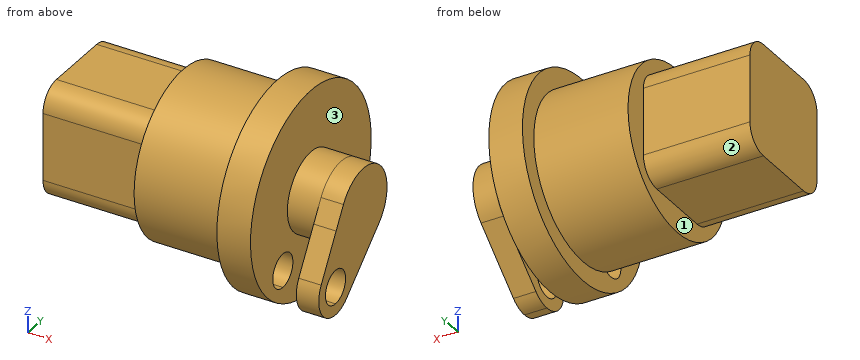
```python
from build123d import *

# Parameters (mm, degrees)
SKETCH2_R           = 9
BOSS_EXTRUDE1_DEPTH = 3
SKETCH2_4_R         = 7.3
BOSS_EXTRUDE2_DEPTH = 8.4
BOSS_EXTRUDE3_START = -8.4
SKETCH2_6_W         = 10
SKETCH2_6_H         = 10
BOSS_EXTRUDE3_DEPTH = 9.5
BOSS_EXTRUDE6_START = 3
SKETCH6_R           = 3.5
BOSS_EXTRUDE6_DEPTH = 2.7
BOSS_EXTRUDE7_START = 5.7
BOSS_EXTRUDE7_DEPTH = 2
CUT_EXTRUDE1_DEPTH  = 3
FILLET1_R           = 2


with BuildPart() as part:
    # Sketch2 → Boss-Extrude1 (new body)
    with BuildSketch(Plane(origin=(0, 0, 0), x_dir=(0, 0, -1), z_dir=(1, 0, 0))):
        Circle(SKETCH2_R)
    extrude(amount=BOSS_EXTRUDE1_DEPTH)

    # Sketch2<4> → Boss-Extrude2 (add)
    with BuildSketch(Plane(origin=(0, 0, 0), x_dir=(0, 0, -1), z_dir=(1, 0, 0))):
        Circle(SKETCH2_4_R)
    extrude(amount=-BOSS_EXTRUDE2_DEPTH)

    # Sketch2<6> → Boss-Extrude3 (add)
    with BuildSketch(Plane(origin=(0, 0, 0), x_dir=(0, 0, -1), z_dir=(1, 0, 0)).offset(BOSS_EXTRUDE3_START)):
        Rectangle(SKETCH2_6_W, SKETCH2_6_H)
    extrude(amount=-BOSS_EXTRUDE3_DEPTH)

    # Sketch6 → Boss-Extrude6 (add)
    with BuildSketch(Plane(origin=(0, 0, 0), x_dir=(0, 0, -1), z_dir=(1, 0, 0)).offset(BOSS_EXTRUDE6_START)):
        with Locations(Location((0, 0, 0), (0, 0, 180))):
            Circle(SKETCH6_R)
    extrude(amount=BOSS_EXTRUDE6_DEPTH)

    # Sketch6<4> → Boss-Extrude7 (add)
    with BuildSketch(Plane(origin=(0, 0, 0), x_dir=(0, 0, -1), z_dir=(1, 0, 0)).offset(BOSS_EXTRUDE7_START)):
        with BuildLine():
            ThreePointArc((6.861759117, -2.533034113), (4.954197643, -1.67824538), (3.064177772, -2.571150439))
            Line((3.064177772, -2.571150439), (3.830222216, -3.213938048))
            ThreePointArc((3.830222216, -3.213938048), (5.492319095, -2.768580532), (6.47928888, -4.178119463))
            ThreePointArc((6.47928888, -4.178119463), (6.388827811, -4.691149678), (6.128355545, -5.142300877))
            Line((6.128355545, -5.142300877), (6.894399988, -5.785088487))
            ThreePointArc((6.894399991, -5.785088484), (7.328520433, -5.033169819), (7.47928888, -4.178119463))
            ThreePointArc((7.47928888, -4.178119463), (7.3198204, -3.29953412), (6.861759117, -2.533034113))
        make_face()
        with BuildLine():
            Line((3.830222216, -3.213938048), (3.064177772, -2.571150439))
            ThreePointArc((3.064177772, -2.571150439), (2.513036454, -4.587507997), (3.6860836, -6.31765682))
            ThreePointArc((3.6860836, -6.31765682), (5.388677416, -6.644371889), (6.894399991, -5.785088484))
            Line((6.894399988, -5.785088487), (6.128355545, -5.142300877))
            ThreePointArc((6.128355545, -5.142300877), (4.015107466, -5.327186128), (3.830222216, -3.213938048))
        make_face()
        with BuildLine():
            ThreePointArc((3.5, 0), (3.288924173, -1.197070502), (2.681155551, -2.249756634))
            Line((2.681155551, -2.249756634), (3.064177772, -2.571150439))
            ThreePointArc((3.064177772, -2.571150439), (4.954197643, -1.67824538), (6.861759117, -2.533034113))
            Line((6.861759117, -2.533034113), (2.635458332, 2.303119489))
            ThreePointArc((2.635458332, 2.303119489), (3.276744128, 1.230019479), (3.5, 0))
        make_face()
        with BuildLine():
            Line((3.064177772, -2.571150439), (2.681155551, -2.249756634))
            ThreePointArc((2.681155551, -2.249756634), (1.479163916, -3.172077255), (0, -3.5))
            Line((0, -3.5), (0, -4.089669185))
            Line((0, -4.089669185), (3.6860836, -6.31765682))
            ThreePointArc((3.6860836, -6.31765682), (2.513036454, -4.587507997), (3.064177772, -2.571150439))
        make_face()
        with BuildLine():
            Line((0, -3.5), (0, 0))
            Line((0, 0), (2.681155551, -2.249756634))
            ThreePointArc((2.681155551, -2.249756634), (3.288924173, -1.197070502), (3.5, 0))
            ThreePointArc((3.5, 0), (3.276744128, 1.230019479), (2.635458332, 2.303119489))
            ThreePointArc((2.635458332, 2.303119489), (-2.681155551, 2.249756634), (-1.810487393, -2.9953523))
            ThreePointArc((-1.810487393, -2.9953523), (-0.939751816, -3.371478389), (0, -3.5))
        make_face()
        with BuildLine():
            Line((2.681155551, -2.249756634), (0, 0))
            Line((0, 0), (0, -3.5))
            ThreePointArc((0, -3.5), (1.479163916, -3.172077255), (2.681155551, -2.249756634))
        make_face()
        with BuildLine():
            Line((0, -4.089669185), (0, -3.5))
            ThreePointArc((0, -3.5), (-0.939751816, -3.371478389), (-1.810487393, -2.9953523))
            Line((-1.810487393, -2.9953523), (0, -4.089669185))
        make_face()
    extrude(amount=BOSS_EXTRUDE7_DEPTH)

    # Sketch6<5> → Cut-Extrude1 (cut)
    with BuildSketch(Plane(origin=(0, 0, 0), x_dir=(0, 0, -1), z_dir=(1, 0, 0))):
        with BuildLine():
            ThreePointArc((6.47928888, -4.178119463), (5.492319095, -2.768580532), (3.830222216, -3.213938048))
            Line((3.830222216, -3.213938048), (6.128355545, -5.142300877))
            ThreePointArc((6.128355545, -5.142300877), (6.388827811, -4.691149678), (6.47928888, -4.178119463))
        make_face()
        with BuildLine():
            Line((6.128355545, -5.142300877), (3.830222216, -3.213938048))
            ThreePointArc((3.830222216, -3.213938048), (4.015107466, -5.327186128), (6.128355545, -5.142300877))
        make_face()
    extrude(amount=CUT_EXTRUDE1_DEPTH, mode=Mode.SUBTRACT)

    # Fillet1
    fillet1_edges = [part.edges().sort_by_distance(p)[0] for p in [
        (-13.15, -5, 5),
        (-13.15, 5, 5),
        (-13.15, 5, -5),
        (-13.15, -5, -5),
    ]]
    fillet(fillet1_edges, radius=FILLET1_R)


solid = part.part
```
Verification items for the finished model (mm, model axes). Face numbers are marked on the shaded views. A direction names the side the tool comes from. Coordinates: 2 decimals unless noted, no trailing zeros. Loops run counter-clockwise (first coordinate to the right, second up) from the corner with the lowest first, then second, coordinate; pieces in that order, holes last. Notation, with made-up numbers: (54, 56.5) -> (70, 56.5) arc R25 ccw to (70, 73.5) -> close; hole circle Ø4 at (-19, 41). An arc over 180 degrees is marked (long way). Answer in a Markdown table with one row per item. Add a question column.
1. Material ranges on probe 1 along Z at (x, y) = (-11, 0.75); probe 2 along X at (y, z) = (-4.5, -1.25); probe 3 along X at (y, z) = (-1.5, 6.75), recorded low to high. Write a range as [from, to].
2. Section check B-B, the plane y = 4.5. Enter the section's corners in (x, z).
3. Access from +Z, -Z, +X, -X, +Y, -Y to the whole of each face (thin tool, end or side, straight path). Record for the marked faces 1, 2 and 3.
4. Section check A-A, the plane x = -8.75. Enter the section's corners in (y, z).
5. Depth check by flat-ended pin: P1, Ø5, axis at x = 3.5, y = 4, coming from the -Z side; P2, Ø5, axis at x = -14, z = -2, coming from the +Y side; P3, Ø1.4, axis at y = -4, z = -5.5, coming from the +X side. Enter the tip coordinate at first touch or a pass-through.
6. Section check C-C, the plane z = 6.5. Enter the section's corners in (x, y), then the cut area to 3 significant figures.
7. Section check D-D, the plane y = 0. Enter the section's corners in (x, z), then the cut area to 3 significant figures.
Derived:
| question | item | result |
|---|---|---|
| 1 | probe 1 | z = [-5, 5] |
| 1 | probe 2 | x = [-17.9, 3], [5.7, 7.7] |
| 1 | probe 3 | x = [-8.4, 3] |
| 2 | outline | (-17.9, -4.32) -> (-8.4, -4.32) -> (-8.4, -5.75) -> (0, -5.75) -> (0, -7.79) -> (3, -7.79) -> (3, 7.79) -> (0, 7.79) -> (0, 5.75) -> (-8.4, 5.75) -> (-8.4, 4.32) -> (-17.9, 4.32) -> close |
| 3 | face 1 | -X |
| 3 | face 2 | -Z, -X, +Y |
| 3 | face 3 | none |
| 4 | outline | (-5, -3) arc R2 ccw to (-3, -5) -> (3, -5) arc R2 ccw to (5, -3) -> (5, 3) arc R2 ccw to (3, 5) -> (-3, 5) arc R2 ccw to (-5, 3) -> close |
| 5 | P1 | stops at z = -8.87 |
| 5 | P2 | stops at y = 5 |
| 5 | P3 | stops at x = 0 |
| 6 | outline | (-8.4, -3.32) -> (0, -3.32) -> (0, -6.22) -> (3, -6.22) -> (3, 6.22) -> (0, 6.22) -> (0, 3.32) -> (-8.4, 3.32) -> close |
| 6 | area | 93.2 mm² |
| 7 | outline | (-17.9, -5) -> (-8.4, -5) -> (-8.4, -7.3) -> (0, -7.3) -> (0, -9) -> (3, -9) -> (3, -3.5) -> (5.7, -3.5) -> (5.7, -4.65) -> (7.7, -4.65) -> (7.7, 3.5) -> (3, 3.5) -> (3, 9) -> (0, 9) -> (0, 7.3) -> (-8.4, 7.3) -> (-8.4, 5) -> (-17.9, 5) -> close |
| 7 | area | 307 mm² |
